```python
from build123d import *

# Parameters (mm, degrees)
SKETCH1_W           = 25
SKETCH1_H           = 25
BOSS_EXTRUDE1_DEPTH = 10
SKETCH3_R           = 11.25
SKETCH3_R_2         = 2
CUT_EXTRUDE1_DEPTH  = 10
FILLET1_R           = 2


with BuildPart() as part:
    # Sketch1 → Boss-Extrude1 (new body)
    with BuildSketch(Plane.XY):
        with Locations((12.5, 12.5)):
            Rectangle(SKETCH1_W, SKETCH1_H)
    extrude(amount=BOSS_EXTRUDE1_DEPTH)

    # Sketch3 → Cut-Extrude1 (cut)
    with BuildSketch(Plane.XY.offset(10)):
        with Locations((12.5, 12.5)):
            Circle(SKETCH3_R)
        with Locations((2.5, 22.5)):
            Circle(SKETCH3_R_2)
        with Locations((2.5, 2.5)):
            Circle(SKETCH3_R_2)
        with Locations((22.5, 2.5)):
            Circle(SKETCH3_R_2)
        with Locations((22.5, 22.5)):
            Circle(SKETCH3_R_2)
    extrude(amount=-CUT_EXTRUDE1_DEPTH, mode=Mode.SUBTRACT)

    # Fillet1
    fillet1_edges = [part.edges().sort_by_distance(p)[0] for p in [
        (0, 25, 5),
        (25, 25, 5),
        (25, 0, 5),
        (0, 0, 5),
    ]]
    fillet(fillet1_edges, radius=FILLET1_R)


solid = part.part
```
Work out the finished part from the listing and answer in its coordinate system (mm). Coordinates: 2 decimals unless noted, no trailing zeros. Order: outer loops, then holes, each group sorted by start corner. A loop starts at its lowest first (then second) coordinate and runs counter-clockwise, first axis right, second up. Notation, with made-up numbers: (67, 6) - (72, 6) arc R20 ccw to (72, 21) - close; hole circle Ø3 at (14.25, 26). An arc over 180 degrees is marked (long way). Answer as a JSON object with one key per item and string values.
1. Find section D-D on y = 2.5. Determine the outline of the cut face in (x, z), plus the area to 3 significant figures.
Output values:
{"outline": "(0, 0) - (0.5, 0) - (0.5, 10) - (0, 10) - close; (4.5, 0) - (7.35, 0) - (7.35, 10) - (4.5, 10) - close; (17.65, 0) - (20.5, 0) - (20.5, 10) - (17.65, 10) - close; (24.5, 0) - (25, 0) - (25, 10) - (24.5, 10) - close", "area": "66.9 mm²"}
2. Find section A-A on x = 12.5. Determine the outline of the cut face in (y, z).
Output values:
{"outline": "(0, 0) - (1.25, 0) - (1.25, 10) - (0, 10) - close; (23.75, 0) - (25, 0) - (25, 10) - (23.75, 10) - close"}
3. Consider line 1 (Y direction, x = 22.5, z = 3.75); line 2 (X direction, y = 3.25, z = 3.5); line 3 (X direction, y = 21, z = 8). Determine where each line is inside the solid, lowest interval first.
Output values:
{"line 1": "y = 0 to 0.5, 4.5 to 7.35, 17.65 to 20.5, 24.5 to 25", "line 2": "x = 0 to 0.65, 4.35 to 6.1, 18.9 to 20.65, 24.35 to 25", "line 3": "x = 0 to 1.18, 3.82 to 5.13, 19.87 to 21.18, 23.82 to 25"}
4. The mould has two halves that part along Y. Classify faces 1 (the face through (0.57, 0.6, 5.07)), 2 (the face through (24.4, 24.43, 5.07)), 3 (the face through (3.572, 5.655, 5.07)): +Y half, -Y half, draft (parallel to the pull), parting line (faces both ways), or undercut.
Output values:
{"face 1": "-Y half", "face 2": "+Y half", "face 3": "undercut"}
5. This flat-tipped pin is pushed along its axis until it touches: P1, Ø1.5, axis at x = 15, y = 3.5, coming from the +Z side. Where does it stop, or does it pass through?
Output values:
{"P1": "passes through"}
6. Find section B-B on z = 4. Determine the outline of the cut face in (x, y).
Output values:
{"outline": "(0, 2) arc R2 ccw to (2, 0) - (23, 0) arc R2 ccw to (25, 2) - (25, 23) arc R2 ccw to (23, 25) - (2, 25) arc R2 ccw to (0, 23) - close; hole circle Ø4 at (2.5, 2.5); hole circle Ø4 at (2.5, 22.5); hole circle Ø22.5 at (12.5, 12.5); hole circle Ø4 at (22.5, 2.5); hole circle Ø4 at (22.5, 22.5)"}
7. Find section C-C on y = 7.75. Determine the outline of the cut face in (x, z), plus the area to 3 significant figures.
Output values:
{"outline": "(0, 0) - (2.3, 0) - (2.3, 10) - (0, 10) - close; (22.7, 0) - (25, 0) - (25, 10) - (22.7, 10) - close", "area": "46.0 mm²"}
